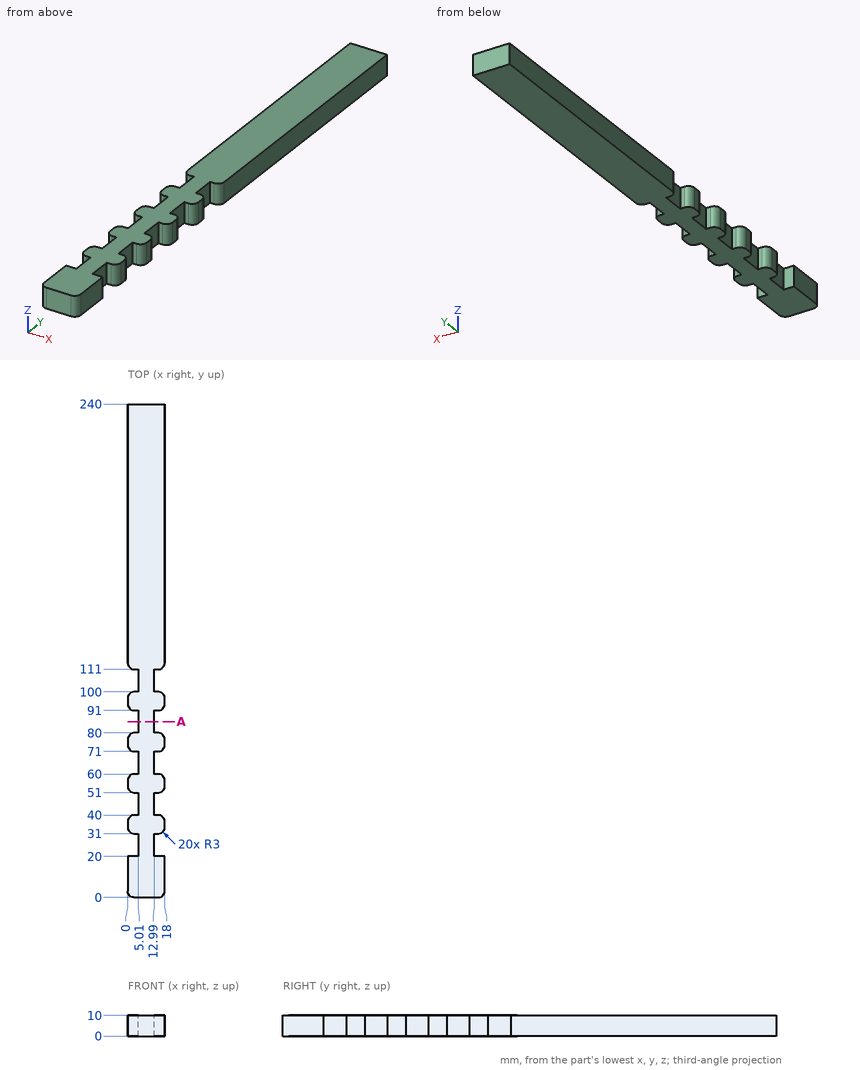
Input: dimensioned drawing with shaded views. Units: mm. Origin: part minimum x, y, z. Round coordinates to 2 decimals unless told otherwise and drop trailing zeros. Order: outer loops, then holes, each group sorted by start corner. A loop starts at its lowest first (then second) coordinate and runs counter-clockwise, first axis right, second up. Notation, with made-up numbers: (-16, -25) - (28, -25) arc R12 ccw to (28, -12) - close; hole circle Ø4 at (9, 20.5). An arc over 180 degrees is marked (long way). Answer as a JSON object with one key per item and string values. Group by question number.
(1) Pin query (flat end, axial travel): P1, Ø5, axis at y = 104, z = 6.5, coming from the -X side; P2, Ø2, axis at y = 31.5, z = 2, coming from the +X side; P3, Ø1.5, axis at y = 60.5, z = 2.5, coming from the -X side. Return the tip coordinate at first contact, or that it passes through.
(2) Cut plane A-A (y = 85.5). Return loops of the section in (x, z), then the cut area to 3 significant figures.
(3) Material intervals for probe 1 along Y at (x, z) = (2.75, 1.25); probe 2 along Y at (x, z) = (17, 3.25); probe 3 along X at (y, z) = (80.5, 3.75), sorted ascending. Write a range as from..to.
Here are the results:
{
 "1": {"P1": "stops at x = 5.01", "P2": "stops at x = 17.6", "P3": "stops at x = 1.8"},
 "2": {"outline": "(5.01, 0) - (12.99, 0) - (12.99, 10) - (5.01, 10) - close", "area": "79.8 mm^2"},
 "3": {"probe 1": "y = 0.01..20, 31.01..39.99, 51.01..59.99, 71.01..79.99, 91.01..99.99, 111.01..240", "probe 2": "y = 0.76..20, 31.76..39.24, 51.76..59.24, 71.76..79.24, 91.76..99.24, 111.76..240", "probe 3": "x = 5.01..12.99"}
}
